from build123d import *

# Parameters (mm, degrees)
BASE_DEPTH              = 3
ESQUISSE2_W             = 20
ESQUISSE2_H             = 20
ENL_V_MAT_EXTRU_1_DEPTH = 4
ESQUISSE4_R             = 2
ENL_V_MAT_EXTRU_4_DEPTH = 3
CONG_1_R                = 3
BOSS_EXTRU_2_DEPTH      = 3
ESQUISSE3_R             = 2.3
TROUS_LIDAR_DEPTH       = 10


with BuildPart() as part:
    # Esquisse1 → Base (new body)
    with BuildSketch(Plane.XY):
        Polygon((0, 0), (-175, 0), (-199.748737342, 24.748737342), (-199.748737342, 284.748737342), (-175, 309.497474683), (0, 309.497474683), (24.748737342, 284.748737342), (24.748737342, 24.748737342), align=None)
    extrude(amount=BASE_DEPTH)

    # Esquisse2 → Enlèv. mat.-Extru.1 (cut, through all)
    with BuildSketch(Plane.XY.offset(3)):
        with Locations((-152.5, 286.497474683)):
            Rectangle(ESQUISSE2_W, ESQUISSE2_H)
        with Locations((-152.5, 23)):
            Rectangle(ESQUISSE2_W, ESQUISSE2_H)
        with Locations((-22.5, 23)):
            Rectangle(ESQUISSE2_W, ESQUISSE2_H)
        with Locations((-22.5, 286.497474683)):
            Rectangle(ESQUISSE2_W, ESQUISSE2_H)
    extrude(amount=-ENL_V_MAT_EXTRU_1_DEPTH, mode=Mode.SUBTRACT)

    # Esquisse4 → Enlèv. mat.-Extru.4 (cut)
    with BuildSketch(Plane.XY.offset(3)):
        with Locations((-152.5, 260.997474683)):
            Circle(ESQUISSE4_R)
        with Locations((-152.5, 48.5)):
            Circle(ESQUISSE4_R)
        with Locations((-22.5, 260.997474683)):
            Circle(ESQUISSE4_R)
        with Locations((-22.5, 48.5)):
            Circle(ESQUISSE4_R)
    extrude(amount=-ENL_V_MAT_EXTRU_4_DEPTH, mode=Mode.SUBTRACT)

    # Congé1
    cong_1_edges = [part.edges().sort_by_distance(p)[0] for p in [
        (0, 0, 1.5),
        (-175, 0, 1.5),
        (-199.748737342, 24.748737342, 1.5),
        (-199.748737342, 284.748737342, 1.5),
        (-175, 309.497474683, 1.5),
        (0, 309.497474683, 1.5),
        (24.748737342, 284.748737342, 1.5),
        (24.748737342, 24.748737342, 1.5),
    ]]
    fillet(cong_1_edges, radius=CONG_1_R)

    # Esquisse6 → Boss.-Extru.2 (add)
    with BuildSketch(Plane.XY.offset(3)):
        Polygon((24.748737342, 214.949513542), (24.748737342, 94.547961141), (24.748737342, 50.529955402), (94.748737342, 94.949513542), (94.748737342, 214.949513542), (24.748737342, 259.369071682), align=None)
    extrude(amount=-BOSS_EXTRU_2_DEPTH)

    # Esquisse3 → trous lidar (cut)
    with BuildSketch(Plane.XY.offset(3)):
        with Locations((-5.251262658, 193.174712193)):
            Circle(ESQUISSE3_R)
        with Locations((55.748737342, 204.174712193)):
            Circle(ESQUISSE3_R)
        with Locations((-5.251262658, 115.174712193)):
            Circle(ESQUISSE3_R)
        with Locations((55.748737342, 104.174712193)):
            Circle(ESQUISSE3_R)
    extrude(amount=-TROUS_LIDAR_DEPTH, mode=Mode.SUBTRACT)


solid = part.part
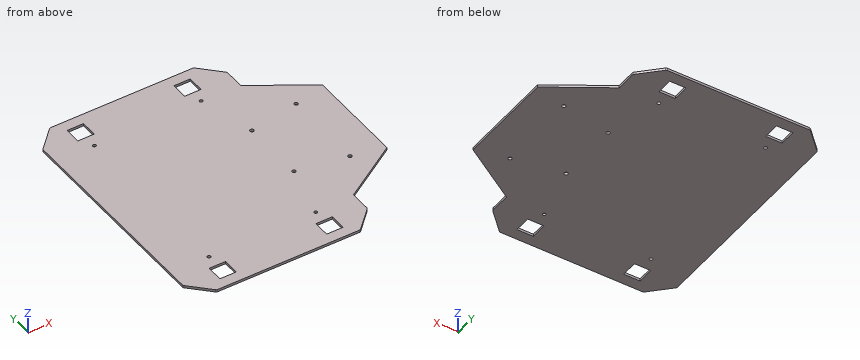
Geometry: final body of the model. Coordinates: model frame, mm. Give positions to 0.01 mm unless a question says otherwise; leave off trailing zeros. Write each loop counter-clockwise with the first axis right and the second up, starting at its lowest first coordinate (ties: lowest second). Pieces come first, ordered by that corner, then holes. Notation, with made-up numbers: (17, 75) - (40, 75) arc R21 cw to (40, 80) - close; hole circle Ø1 at (23, 19.25). An arc over 180 degrees is marked (long way). Return JSON: item names as keys, results as strings. Group by question number.
1) Section B-B on y = 42. Return the cut outline in (x, z), plus the area to 3 significant figures.
2) Section C-C on x = 75. Return the cut outline in (y, z).
3) Section A-A on z = 2.5. State how many separate pieces and enclosed holes the cut face has, plus the area to 3 significant figures.
4) First-contact query: P1, Ø1.5, axis at y = 289.5, z = 1.5, coming from the +X side; P2, Ø1.5, axis at y = 19, z = 2, coming from the +X side; P3, Ø0.9, axis at y = 286, z = 1.5, coming from the -X side. Flat tips, straight axial feed; report the tip coordinate or a pass-through.
5) Line query: line 1 (X direction, y = 49, z = 2.3); line 2 (Y direction, x = -158.5, z = 1.5); line 3 (X direction, y = 27, z = 1.15). Output: solid intervals per line, ascending.
Filled in:
{
 "1": {"outline": "(-199.75, 0) - (24.75, 0) - (24.75, 3) - (-199.75, 3) - close", "area": "673 mm^2"},
 "2": {"outline": "(82.42, 0) - (227.48, 0) - (227.48, 3) - (82.42, 3) - close"},
 "3": {"separate pieces": "1", "enclosed holes": "12", "area": "78,000 mm^2"},
 "4": {"P1": "stops at x = 20.75", "P2": "stops at x = 19.75", "P3": "stops at x = -198.94"},
 "5": {"line 1": "x = -199.75 to -154.44, -150.56 to -24.44, -20.56 to 24.75", "line 2": "y = 0 to 13, 33 to 276.5, 296.5 to 309.5", "line 3": "x = -199.75 to -162.5, -142.5 to -32.5, -12.5 to 24.75"}
}
